Job drawing, mm, ordinate dimensions from the low corner. One solid piece. A direction names the side the tool comes from. Give positions to 0.01 mm unless a question says otherwise; leave off trailing zeros. Loops run counter-clockwise (first coordinate to the right, second up) from the corner with the lowest first, then second, coordinate; pieces in that order, holes last.
Item 1: Probe probe 1 along X at (y, z) = (20.5, 24); probe 2 along X at (y, z) = (5.5, 10.5); probe 3 along Y at (x, z) = (30, 22). List the from-to ranges inside material, lowest first.
Item 2: Saw through at C-C on z = 5.5. Give the cut face in (x, y).
Item 3: Drop flat-ended pins along their axis: P1, Ø7.5, axis at y = 17.5, z = 9.5, coming from the +X side; P2, Ø8, axis at x = 8, z = 23, coming from the -Y side; P3, Ø5, axis at x = 18.542, z = 15.875, coming from the -Y side; P4, Ø4, axis at x = 77.5, y = 3.5, coming from the +Z side. Give the stop position or say it passes through.
Item 4: Saw through at D-D on y = 22.5. Give the cut face in (x, z) (3 decimals), plus the area to 3 significant figures.
Item 5: Saw through at A-A on y = 11. Give the cut face in (x, z), plus the area to 3 significant figures.
Item 6: Mould opens along Y. For the marked faces 1, 2 and 3 say: released by +Y, released by -Y, zero draft, split by the parting line, or undercut.
Item 7: Which spindle directions (+Z, -Z, +X, -X, +Y, -Y) get a long thin tool onto all of the face, cutting with end or side? Do the marked faces 4, 5 and 6. Say none if no direction does.
Item 8: Saw through at B-B on z = 14. Give the cut face in (x, y), plus the area to 3 significant figures.
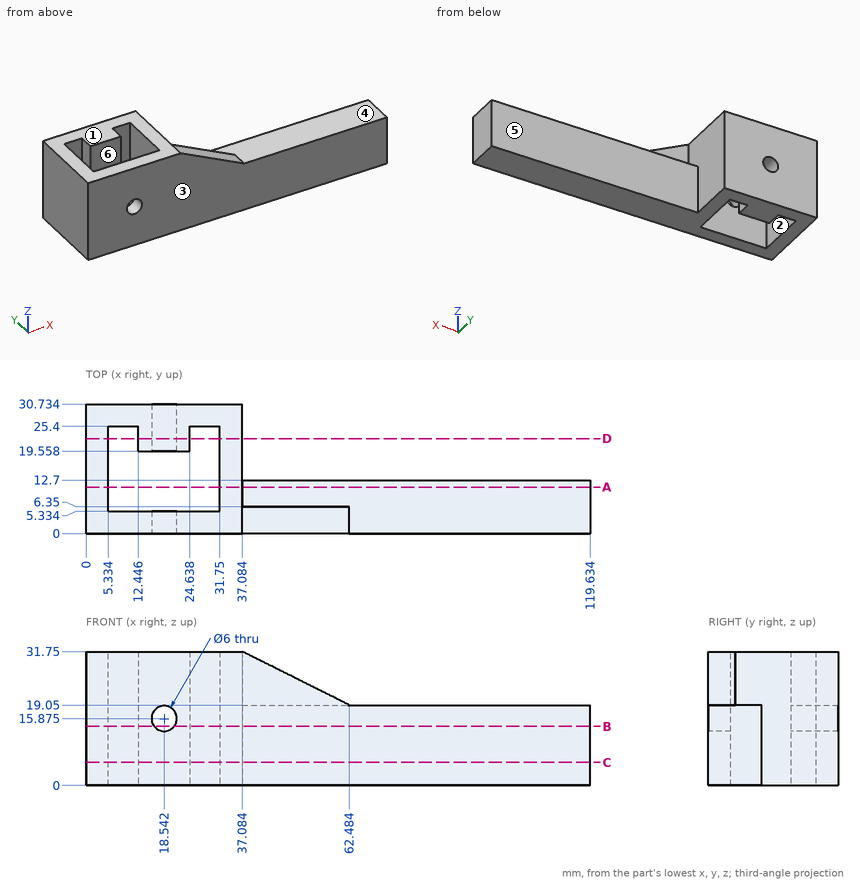
Results below:
1. probe 1: x = 0 to 5.33, 12.45 to 24.64, 31.75 to 37.08
1. probe 2: x = 0 to 5.33, 31.75 to 119.63
1. probe 3: y = 0 to 5.33, 25.4 to 30.73
2. outline: (0, 0) - (119.63, 0) - (119.63, 12.7) - (37.08, 12.7) - (37.08, 30.73) - (0, 30.73) - close; hole (5.33, 5.33) - (31.75, 5.33) - (31.75, 25.4) - (24.64, 25.4) - (24.64, 19.56) - (12.45, 19.56) - (12.45, 25.4) - (5.33, 25.4) - close
3. P1: stops at x = 37.08
3. P2: stops at y = 0
3. P3: passes through
3. P4: stops at z = 19.05
4. outline: (0, 0) - (5.334, 0) - (5.334, 31.75) - (0, 31.75) - close; (12.446, 0) - (24.638, 0) - (24.638, 31.75) - (12.446, 31.75) - close; (31.75, 0) - (37.084, 0) - (37.084, 31.75) - (31.75, 31.75) - close; hole circle Ø6 at (18.542, 15.875)
4. area: 698 mm2
5. outline: (0, 0) - (5.33, 0) - (5.33, 31.75) - (0, 31.75) - close; (31.75, 0) - (119.63, 0) - (119.63, 19.05) - (37.08, 19.05) - (37.08, 31.75) - (31.75, 31.75) - close
5. area: 1,910 mm2
6. face 1: zero draft
6. face 2: undercut
6. face 3: released by -Y
7. face 4: +Z, +X, +Y
7. face 5: +Z, -Z, +X, +Y
7. face 6: +Z, -Z
8. outline: (0, 0) - (16.2, 0) - (16.2, 5.33) - (5.33, 5.33) - (5.33, 25.4) - (12.45, 25.4) - (12.45, 19.56) - (16.2, 19.56) - (16.2, 30.73) - (0, 30.73) - close; (20.88, 0) - (119.63, 0) - (119.63, 12.7) - (37.08, 12.7) - (37.08, 30.73) - (20.88, 30.73) - (20.88, 19.56) - (24.64, 19.56) - (24.64, 25.4) - (31.75, 25.4) - (31.75, 5.33) - (20.88, 5.33) - close
8. area: 1,650 mm2
